from build123d import *

# Parameters (mm, degrees)
F0_W     = 41.4018779993
F0_H     = 24.4389437139
F1_DEPTH = 25
F4_R     = 3.5686331082
F6_R     = 5


with BuildPart() as f1:
    # F0 (on Front) → F1 (new body)
    with BuildSketch(Plane.XZ):
        with Locations((20.7009389997, 12.219471857)):
            Rectangle(F0_W, F0_H)
    extrude(amount=F1_DEPTH)

    # F5: sweep along a path in F3
    with BuildLine(Plane.XZ.offset(12.5)) as f5_path:
        Line((19.1687617356, 24.4389437139), (19.1687617356, 16.1529793682))
        ThreePointArc((19.1687617356, 16.1529793682), (21.1352572497, 11.4054392279), (25.88279739, 9.4389437139))
        Line((25.88279739, 9.4389437139), (41.4018779993, 9.4389437139))
    # F4 (on face) → F5 (sweep, cut)
    with BuildSketch(Plane.YZ.offset(41.4018779993)):
        with Locations((-12.5, 9.4434265047)):
            Circle(F4_R)
    sweep(path=f5_path.line, mode=Mode.SUBTRACT)

    # F6
    f6_edges = [f1.edges().sort_by_distance(p)[0] for p in [
        (41.401878, 0, 12.219472),
        (20.700939, 0, 24.438944),
        (0, 0, 12.219472),
        (20.700939, 0, 0),
        (41.401878, -25, 12.219472),
        (20.700939, -25, 24.438944),
        (0, -25, 12.219472),
        (20.700939, -25, 0),
        (41.401878, -12.5, 0),
        (0, -12.5, 0),
        (41.401878, -12.5, 24.438944),
        (0, -12.5, 24.438944),
    ]]
    fillet(f6_edges, radius=F6_R)


solid = f1.part
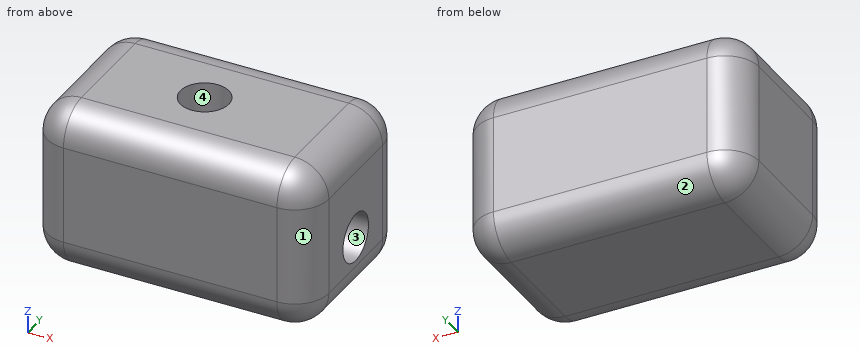
Geometry check sheet. Reference: the model listing, model coordinates, mm. Face numbers are marked on the shaded views. Give positions to 0.01 mm unless a question says otherwise; leave off trailing zeros. Order: outer loops, then holes, each group sorted by start corner. A loop starts at its lowest first (then second) coordinate and runs counter-clockwise, first axis right, second up. Notation, with made-up numbers: (37, -34.5) - (42, -34.5) arc R30 ccw to (42, -11.5) - close; hole circle Ø2 at (27.25, -24). An arc over 180 degrees is marked (long way). Use one line per item in the form item = value.
1) Sectioned sample at C-C (z = 17.75). Record the boundary of the cut face in (x, y).
Working result:
outline = (0, -20) arc R5 ccw to (5, -25) - (36.4, -25) arc R5 ccw to (41.4, -20) - (41.4, -5) arc R5 ccw to (36.4, 0) - (5, 0) arc R5 ccw to (0, -5) - close; hole circle Ø7.14 at (19.17, -12.5)
2) Sectioned sample at B-B (x = 10.5). Record the boundary of the cut face in (y, z).
Working result:
outline = (-25, 5) arc R5 ccw to (-20, 0) - (-5, 0) arc R5 ccw to (0, 5) - (0, 19.44) arc R5 ccw to (-5, 24.44) - (-20, 24.44) arc R5 ccw to (-25, 19.44) - close
3) Material ranges on probe 1 along Z at (x, y) = (32, -12.5); probe 2 along X at (y, z) = (-12.5, 18.75); probe 3 along Y at (x, z) = (18, 22.25), recorded low to high. Write a range as from..to.
Working result:
probe_1 = 0..5.87, 13.01..24.44
probe_2 = 0..15.6, 22.74..41.4
probe_3 = -24.13..-15.87, -9.13..-0.87
4) Draft check along Y on the marked faces 1, 2, 3 and 4. Enter one of: released by +Y, released by -Y, zero draft, split by the parting line, or undercut.
Working result:
face_1 = released by -Y
face_2 = released by +Y
face_3 = undercut
face_4 = undercut
5) Depth check by flat-ended pin: pin 1 Ø8 at (y, z) = (-3.5, 5) entering from -X. Enter the tip coordinate at first touch or a pass-through.
Working result:
pin_1 = 0
6) Sectioned sample at D-D (y = -2.5). Record the boundary of the cut face in (x, z), and give its area (3 significant figures).
Working result:
outline = (0.67, 5) arc R4.33 ccw to (5, 0.67) - (36.4, 0.67) arc R4.33 ccw to (40.73, 5) - (40.73, 19.44) arc R4.33 ccw to (36.4, 23.77) - (5, 23.77) arc R4.33 ccw to (0.67, 19.44) - close
area = 909 mm^2
7) Sectioned sample at A-A (y = -12.5). Record the boundary of the cut face in (x, z).
Working result:
outline = (0, 5) arc R5 ccw to (5, 0) - (36.4, 0) arc R5 ccw to (41.4, 5) - (41.4, 5.87) - (25.88, 5.87) arc R10.28 cw to (15.6, 16.15) - (15.6, 24.44) - (5, 24.44) arc R5 ccw to (0, 19.44) - close; (22.74, 16.15) arc R3.14 ccw to (25.88, 13.01) - (41.4, 13.01) - (41.4, 19.44) arc R5 ccw to (36.4, 24.44) - (22.74, 24.44) - close
